Autodesk Inventor part; units mm, degrees
ref_plane "YZ Plane" through (0, 0, 0) normal (1, 0, 0) x (0, 1, 0)
ref_plane "XZ Plane" through (0, 0, 0) normal (0, 1, 0) x (-1, 0, 0)
ref_plane "XY Plane" through (0, 0, 0) normal (0, 0, 1) x (1, 0, 0)
sketch "Sketch1" plane through (0, 0, 0) normal (0, 1, 0) x (-1, 0, 0)
  circle A0 centre (0, 0) radius 2.5
  circle A1 centre (0, 0) radius 4
  dimension "d228" = 5
  dimension "d229" = 8
extrude "Extrusion1" add sketch "Sketch1" against normal blind 30 contours A0
extrude "Extrusion2" add sketch "Sketch1" along normal blind 2 contours A0 | A1
fillet "Fillet1" radius 0.5 1 edges at (4, 2, 0)
sketch "Sketch2" plane through (0, 2, 0) normal (0, 1, 0) x (1, 0, 0)
  line L0 (0.75, -4) -> (-0.75, -4)
  line L1 (-0.75, -4) -> (-0.75, 4)
  line L2 (-0.75, 4) -> (0.75, 4)
  line L3 (0.75, 4) -> (0.75, -4)
  circle A0 centre (0, 0) radius 4
  line L4 (0, -4) -> (0, 4)
  line L5 (-2.5, -0.5) -> (2.5, -0.5)
  line L6 (2.5, -0.5) -> (2.5, 0.5)
  line L7 (2.5, 0.5) -> (-2.5, 0.5)
  line L8 (-2.5, 0.5) -> (-2.5, -0.5)
  line L9 (-4, 0) -> (4, 0)
  line L10 (-0.75, -2.5) -> (0.75, -2.5)
  line L11 (0.75, -2.5) -> (0.75, 2.5)
  line L12 (0.75, 2.5) -> (-0.75, 2.5)
  line L13 (-0.75, 2.5) -> (-0.75, -2.5)
  line L14 (-0.5, 0.5) -> (0.5, 0.5)
  line L15 (0.5, 0.5) -> (0.5, -0.5)
  line L16 (0.5, -0.5) -> (-0.5, -0.5)
  line L17 (-0.5, -0.5) -> (-0.5, 0.5)
  point P0 (-0.75, -3.9291)
  point P1 (0.75, -3.9291)
  point P2 (0.75, 3.9291)
  point P3 (-0.75, 3.9291)
  point P4 (0.75, 0.5)
  point P5 (-0.75, 0.5)
  point P6 (-0.75, -0.5)
  point P7 (0.75, -0.5)
  dimension "d234" = 8
  dimension "d235" = 1.5
  dimension "d236" = 1
  dimension "d237" = 5
  dimension "d238" = 5
  dimension "d243" = 1
  dimension "d244" = 1
extrude "Extrusion3" cut sketch "Sketch2" against normal blind 2 contours L5 L17 L9 L4 | L4 L9 L15 L5 | L9 L17 L7 L4 | L4 L7 L15 L9
chamfer "Chamfer1" distance 2 angle 45 4 edges at (-0.5, 2, 0) (0.5, 2, 0) (0, 2, 0.5) (0, 2, -0.5)
extrude "Extrusion4" cut sketch "Sketch2" against normal blind 1 contours L4 L10 L3 A0 | A0 L1 L10 L4 | L10 L1 L5 L4 | L4 L5 L3 L10 | L3 L12 L4 A0 | A0 L4 L12 L1 | L3 L7 L4 L12 | L12 L4 L7 L1
extrude "Extrusion5" add sketch "Sketch2" against normal blind 2 contours L3 L5 L6 L9 A0 | A0 L9 L8 L5 L1 | L9 L6 L7 L3 A0 | A0 L1 L7 L8 L9
thread "Thread1"
fillet "Fillet2" radius 1 2 edges at (4, 2, 0) (-4, 2, 0)
fillet "Fillet3" radius 0.5 4 edges at (-0.75, 1.125, -0.5) (0.75, 1.125, -0.5) (-0.75, 1.125, 0.5) (0.75, 1.125, 0.5)
properties part number "Langbektang houder" material "Steel, Mild"
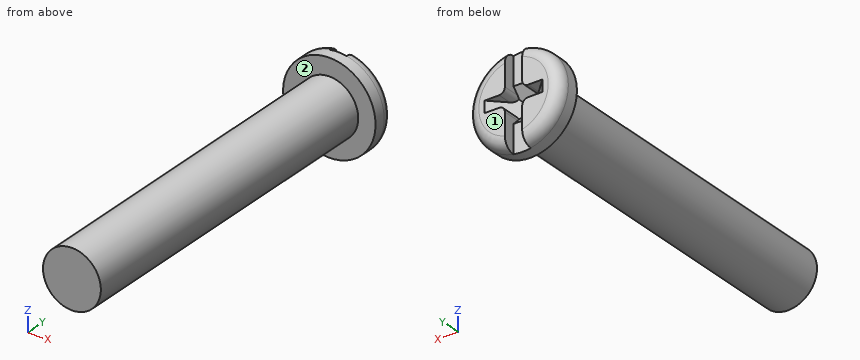
Source: CAD feature listing. Evaluate the final solid. Frame: model axes, mm. Face numbers are marked on the shaded views. A direction names the side the tool comes from. Give positions to 0.01 mm unless a question says otherwise; leave off trailing zeros. Write each loop counter-clockwise with the first axis right and the second up, starting at its lowest first coordinate (ties: lowest second). Pieces come first, ordered by that corner, then holes. Notation, with made-up numbers: (37.5, 13.25) -> (83.5, 13.25) arc R17 cw to (83.5, 24.25) -> close; hole circle Ø3 at (79.5, 69.25). An arc over 180 degrees is marked (long way). Write item = value, one per line.
Q1. First-contact query: pin 1 (4 mm diameter, centred on y = -22.5, z = -2, fed in from -X); pin 2 (0.6 mm diameter, centred on x = 2, y = 1.5, fed in from +Z); pin 3 (1.2 mm diameter, centred on y = 1.5, z = -3, fed in from +X). Flat tips, straight axial feed; report the tip coordinate or a pass-through.
Here are the results:
pin_1 = -2.5
pin_2 = 3.53
pin_3 = 3.12
Q2. Reachability of the marked faces 1 and 2 from +Z, -Z, +X, -X, +Y, -Y: full face, straight path, thin tool, end or side. Return the list, or none.
Here are the results:
face_1 = +Z, -Z, +X, -X, +Y
face_2 = -Y
Q3. Cut plane A-A on z = 0. Return loops of the section in (x, y), then the cut area to 3 significant figures.
Here are the results:
outline = (-4, 0) -> (-2.5, 0) -> (-2.5, -30) -> (2.5, -30) -> (2.5, 0) -> (4, 0) -> (4, 1) arc R1 ccw to (3, 2) -> (2.5, 2) -> (0.5, 0) -> (-0.5, 0) -> (-2.5, 2) -> (-3, 2) arc R1 ccw to (-4, 1) -> close
area = 160 mm²
Q4. Cut plane B-B on x = 0. Return loops of the section in (y, z), then the cut area to 3 significant figures.
Here are the results:
outline = (-30, -2.5) -> (0, -2.5) -> (0, -4) -> (1, -4) -> (1, -1.5) -> (0, -0.5) -> (0, 0.5) -> (1, 1.5) -> (1, 4) -> (0, 4) -> (0, 2.5) -> (-30, 2.5) -> close
area = 156 mm²
Q5. Cut plane C-C on y = -13.5. Return loops of the section in (x, z).
Here are the results:
outline = circle Ø5 at (0, 0)
Q6. Line query: line 1 (Z direction, x = -2, y = -1); line 2 (Y direction, x = 0.5, z = -3). Output: solid intervals per line, ascending. Write a range as from..to.
Here are the results:
line_1 = -1.5..1.5
line_2 = 0..1
